Read the model definition and answer for the solid it produces. Units are mm, in the model's axes. A direction names the side the tool comes from. Coordinates: 2 decimals unless noted, no trailing zeros. Write each loop counter-clockwise with the first axis right and the second up, starting at its lowest first coordinate (ties: lowest second). Pieces come first, ordered by that corner, then holes. Notation, with made-up numbers: (68.25, 86) -> (102.25, 86) arc R26 cw to (102.25, 112) -> close; hole circle Ø5 at (-21, 67.25). An arc over 180 degrees is marked (long way). Use CSV: the item, a comma, the result in double quotes.
from build123d import *

# Parameters (mm, degrees)
SKETCH_1_W       = 103
SKETCH_1_H       = 82
SKETCH_1_W_2     = 95
SKETCH_1_H_2     = 76
EXTRUDE_2_DEPTH  = 2
EXTRUDE_3_DEPTH  = 4
EXTRUDE_4_DEPTH  = 4
EXTRUDE_5_DEPTH  = 4
EXTRUDE_6_DEPTH  = 4
EXTRUDE_7_DEPTH  = 4
EXTRUDE_8_DEPTH  = 4
EXTRUDE_9_DEPTH  = 4
EXTRUDE_10_DEPTH = 4


with BuildPart() as part:
    # Эскиз1 → Бобышка-Вытянуть2 (new body)
    with BuildSketch(Plane(origin=(0, 0, 0), x_dir=(1, 0, 0), z_dir=(0, 1, 0))):
        Rectangle(SKETCH_1_W, SKETCH_1_H)
        Rectangle(SKETCH_1_W_2, SKETCH_1_H_2, mode=Mode.SUBTRACT)
    extrude(amount=EXTRUDE_2_DEPTH)

    # Эскиз6 → Бобышка-Вытянуть3 (add)
    with BuildSketch(Plane(origin=(51.5, 0, 0), x_dir=(0, 0, -1), z_dir=(1, 0, 0))):
        Polygon((31, 2), (36, 2), (36, 5.4), align=None)
        Polygon((36, 2), (41, 2), (41, 8), (36, 8), (36, 6.5), (39, 6.5), (39, 5.4), (36, 5.4), align=None)
    extrude(amount=-EXTRUDE_3_DEPTH)

    # Эскиз7 → Бобышка-Вытянуть4 (add)
    with BuildSketch(Plane(origin=(51.5, 0, 0), x_dir=(0, 0, -1), z_dir=(1, 0, 0))):
        Polygon((-41, 8), (-41, 2), (-36, 2), (-36, 5.4), (-39, 5.4), (-39, 6.5), (-36, 6.5), (-36, 8), align=None)
        Polygon((-36, 5.4), (-36, 2), (-31, 2), align=None)
    extrude(amount=-EXTRUDE_4_DEPTH)

    # Эскиз9 → Бобышка-Вытянуть5 (add)
    with BuildSketch(Plane.ZY.offset(51.5)):
        Polygon((-41, 8), (-41, 2), (-36, 2), (-36, 5.4), (-39, 5.4), (-39, 6.5), (-36, 6.5), (-36, 8), align=None)
        Polygon((-36, 5.4), (-36, 2), (-31, 2), align=None)
    extrude(amount=-EXTRUDE_5_DEPTH)

    # Эскиз10 → Бобышка-Вытянуть6 (add)
    with BuildSketch(Plane.ZY.offset(51.5)):
        Polygon((36, 2), (41, 2), (41, 8), (36, 8), (36, 6.5), (39, 6.5), (39, 5.4), (36, 5.4), align=None)
        Polygon((31, 2), (36, 2), (36, 5.4), align=None)
    extrude(amount=-EXTRUDE_6_DEPTH)

    # Эскиз11 → Бобышка-Вытянуть7 (add)
    with BuildSketch(Plane.XY.offset(41)):
        Polygon((-47.5, 2), (-47.5, 5.4), (-42.5, 2), align=None)
    extrude(amount=-EXTRUDE_7_DEPTH)

    # Эскиз12 → Бобышка-Вытянуть8 (add)
    with BuildSketch(Plane.XY.offset(41)):
        Polygon((47.5, 2), (47.5, 5.4), (42.5, 2), align=None)
    extrude(amount=-EXTRUDE_8_DEPTH)

    # Эскиз13 → Бобышка-Вытянуть9 (add)
    with BuildSketch(Plane(origin=(0, 0, -41), x_dir=(-1, 0, 0), z_dir=(0, 0, -1))):
        Polygon((-47.5, 2), (-47.5, 5.4), (-42.5, 2), align=None)
    extrude(amount=-EXTRUDE_9_DEPTH)

    # Эскиз14 → Бобышка-Вытянуть10 (add)
    with BuildSketch(Plane(origin=(0, 0, -41), x_dir=(-1, 0, 0), z_dir=(0, 0, -1))):
        Polygon((47.5, 2), (47.5, 5.4), (42.5, 2), align=None)
    extrude(amount=-EXTRUDE_10_DEPTH)


solid = part.part
1. Each of these flat-tipped pins is pushed along its axis until it touches: pin 1 Ø1.5 at (x, z) = (-49, 37.5) entering from -Y; pin 2 Ø1.5 at (x, z) = (-10, 39) entering from +Y. Where does it stop, or does it pass through?
Solutions:
pin 1,"stops at y = 0"
pin 2,"stops at y = 2"
2. A cutting plane is placed at A-A (x = -13). Give the vertices of the cut face in (y, z), and give its area (3 significant figures).
Solutions:
outline,"(0, -41) -> (2, -41) -> (2, -38) -> (0, -38) -> close; (0, 38) -> (2, 38) -> (2, 41) -> (0, 41) -> close"
area,"12.0 mm^2"
3. For a pull along Z with two mould halves and no side action, classify faces 5 (the flat face through (-50, 5.4, -37)), 6 (the flat face through (50, 8, -39)), 7 (the flat face through (0, 1, -41)) as pulls with the +Z half, pulls with the -Z half, needs draft (parallel to the pull), parting line crosses it, or undercut.
Solutions:
face 5,"undercut"
face 6,"needs draft"
face 7,"pulls with the -Z half"
4. A tool of negligible diameter and unlimited length cuts with its end or side. For faces 1 (the flat face through (47.5, 7, -39)), 2 (the flat face through (-46, 3, 37)), 3 (the flat face through (50, 6.5, 38)), 4 (the flat face through (49.5, 3.7, -33.5)), from which of +Z, -Z, +X, -X, +Y, -Y can it reach the whole face along a straight path? Write none if from no direction.
Solutions:
face 1,"+Z, -Z, +Y"
face 2,"+Y, -Y"
face 3,"+X, -X"
face 4,"+X, -X, +Y"
5. Find the intervals of material crossed by line 1 along X through (y, z) = (0.5, 30); line 2 along Z through (x, y) = (-46, 2.75), in increasing order.
Solutions:
line 1,"x = -51.5 to -47.5, 47.5 to 51.5"
line 2,"z = -41 to -37, 37 to 41"
6. A cutting plane is placed at B-B (z = 33.5). Give the vertices of the cut face in (x, y), and give its area (3 significant figures).
Solutions:
outline,"(-51.5, 0) -> (-47.5, 0) -> (-47.5, 3.7) -> (-51.5, 3.7) -> close; (47.5, 0) -> (51.5, 0) -> (51.5, 3.7) -> (47.5, 3.7) -> close"
area,"29.6 mm^2"
7. A cutting plane is placed at C-C (y = 3.75). Give the vertices of the cut face in (x, z), and give its area (3 significant figures).
Solutions:
outline,"(-51.5, -41) -> (-45.07, -41) -> (-45.07, -37) -> (-47.5, -37) -> (-47.5, -33.57) -> (-51.5, -33.57) -> close; (-51.5, 33.57) -> (-47.5, 33.57) -> (-47.5, 37) -> (-45.07, 37) -> (-45.07, 41) -> (-51.5, 41) -> close; (45.07, -41) -> (51.5, -41) -> (51.5, -33.57) -> (47.5, -33.57) -> (47.5, -37) -> (45.07, -37) -> close; (45.07, 37) -> (47.5, 37) -> (47.5, 33.57) -> (51.5, 33.57) -> (51.5, 41) -> (45.07, 41) -> close"
area,"158 mm^2"
